```python
from build123d import *

# Parameters (mm, degrees)
BOSS_EXTRUDE1_DEPTH = 3
FILLET1_R           = 3
FILLET2_R           = 5
FILLET3_R           = 4
FILLET4_R           = 1
FILLET5_R           = 10


with BuildPart() as part:
    # Sketch2 → Boss-Extrude1 (new body)
    with BuildSketch(Plane(origin=(0, 0, 0), x_dir=(1, 0, 0), z_dir=(0, 1, 0))):
        with BuildLine():
            Line((104.861742338, 51.61), (96.285742338, 51.61))
            ThreePointArc((96.285742338, 51.61), (94.785742338, 50.11), (96.285742338, 48.61))
            Line((96.285742338, 48.61), (104.861742338, 48.61))
            Line((104.861742338, 48.61), (104.861742338, 42.36))
            Line((104.861742338, 42.36), (101.159535482, 30.341590159))
            ThreePointArc((101.159535482, 30.341590159), (102.15147179, 28.466473533), (104.026588416, 29.458409841))
            Line((104.026588416, 29.458409841), (107.0705594, 39.34))
            ThreePointArc((107.0705594, 39.34), (110.559148386, 33.719570051), (111.09, 27.125809175))
            Line((111.09, 27.125809175), (105.531161353, 18.360668643))
            ThreePointArc((105.531161353, 18.360668643), (84.319857644, 28.006827284), (67.651742338, 44.29))
            Line((67.651742338, 44.29), (61.935762488, 23.027584397))
            Line((61.935762488, 23.027584397), (57.13, 16.32))
            Line((57.13, 16.32), (49.95, 19.39))
            Line((49.95, 19.39), (25.830040494, 11.99))
            ThreePointArc((25.830040494, 11.99), (24.800734775, 10.253880031), (26.431506195, 9.064692331))
            ThreePointArc((26.431506195, 9.064692331), (36.664028635, 8.803570476), (46.46571567, 5.854056721))
            Line((46.46571567, 5.854056721), (45.9, 1.991540554))
            Line((45.9, 1.991540554), (41.660045255, 2.482673431))
            Line((41.660045255, 2.482673431), (38.9, -1.2))
            Line((38.9, -1.2), (27.015518097, 3.924692331))
            Line((27.015518097, 3.924692331), (20.16, 0))
            Line((20.16, 0), (0, 0))
            Line((0, 0), (0, 4.28))
            Line((0, 4.28), (8.255364291, 5.2))
            ThreePointArc((8.255364291, 5.2), (9.58, 6.856906829), (7.923093171, 8.181542538))
            Line((7.923093171, 8.181542538), (-3.121398875, 6.950714639))
            Line((-3.121398875, 6.950714639), (-7.499203077, 8.482641989))
            Line((-7.499203077, 8.482641989), (-11.827625236, 7.22158903))
            Line((-11.827625236, 7.22158903), (-19.255161489, 11.297641869))
            Line((-19.255161489, 11.297641869), (-23.205269456, 10.857431213))
            Line((-23.205269456, 10.857431213), (-22.269740859, 7.646334739))
            Line((-22.269740859, 7.646334739), (-24.812537217, 7.22158903))
            ThreePointArc((-24.812537217, 7.22158903), (-27.256062178, 10.796585791), (-27.5, 15.12))
            ThreePointArc((-27.5, 15.12), (-22.484233626, 16.792009689), (-17.704912147, 14.531121607))
            ThreePointArc((-17.704912147, 14.531121607), (-4.702395419, 12.521774189), (8.186937419, 15.161474421))
            Line((8.186937419, 15.161474421), (21.991482078, 21.019847276))
            Line((21.991482078, 21.019847276), (29.148159429, 28.986869108))
            Line((29.148159429, 28.986869108), (36.03, 31.378427725))
            Line((36.03, 31.378427725), (41.652863678, 73.662098134))
            ThreePointArc((41.652863678, 73.662098134), (47.001876481, 83.094401265), (57.4, 86.17))
            Line((57.4, 86.17), (89.772823478, 69.836247096))
            ThreePointArc((89.772823478, 69.836247096), (90.799785464, 67.40403524), (93.25912827, 66.443859006))
            ThreePointArc((93.25912827, 66.443859006), (102.166931279, 63.469413825), (107.0705594, 55.46))
            Line((107.0705594, 55.46), (104.861742338, 51.61))
        make_face()
    extrude(amount=BOSS_EXTRUDE1_DEPTH)

    # Fillet1
    fillet1_edges = [part.edges().sort_by_distance(p)[0] for p in [
        (46.46571567, 1.5, -5.854056721),
        (38.9, 1.5, 1.2),
        (20.16, 1.5, 0),
        (-27.5, 1.5, -15.12),
        (29.148159429, 1.5, -28.986869108),
        (89.772823478, 1.5, -69.836247096),
    ]]
    fillet(fillet1_edges, radius=FILLET1_R)

    # Fillet2
    fillet2_edges = [part.edges().sort_by_distance(p)[0] for p in [
        (104.861742338, 1.5, -42.36),
        (111.09, 1.5, -27.125809175),
        (105.531161353, 1.5, -18.360668643),
        (61.935762488, 1.5, -23.027584397),
        (49.95, 1.5, -19.39),
        (27.015518097, 1.5, -3.924692331),
    ]]
    fillet(fillet2_edges, radius=FILLET2_R)

    # Fillet3
    fillet3_edges = [part.edges().sort_by_distance(p)[0] for p in [
        (57.13, 1.5, -16.32),
        (-3.121398875, 1.5, -6.950714639),
        (-7.499203077, 1.5, -8.482641989),
        (-11.827625236, 1.5, -7.22158903),
        (-19.255161489, 1.5, -11.297641869),
        (36.03, 1.5, -31.378427725),
    ]]
    fillet(fillet3_edges, radius=FILLET3_R)

    # Fillet4
    fillet4_edges = [part.edges().sort_by_distance(p)[0] for p in [
        (45.9, 1.5, -1.991540554),
        (0, 1.5, 0),
        (-23.205269456, 1.5, -10.857431213),
        (-22.269740859, 1.5, -7.646334739),
        (-24.812537217, 1.5, -7.22158903),
    ]]
    fillet(fillet4_edges, radius=FILLET4_R)

    # Fillet5
    fillet5_edges = [part.edges().sort_by_distance(p)[0] for p in [
        (57.4, 1.5, -86.17),
    ]]
    fillet(fillet5_edges, radius=FILLET5_R)


solid = part.part
```
Input: part model. Units: mm. Frame: model coordinates. A direction names the side the tool comes from. Coordinates: 2 decimals unless noted, no trailing zeros. Write each loop counter-clockwise with the first axis right and the second up, starting at its lowest first coordinate (ties: lowest second). Pieces come first, ordered by that corner, then holes. Notation, with made-up numbers: (55.25, 28.5) -> (74.25, 28.5) arc R7 cw to (74.25, 37.5) -> close; hole circle Ø5 at (62, 47). An arc over 180 degrees is marked (long way). Answer as a JSON object with one key per item and string values.
1. Mould query, pull axis Z, two halves, no side actions, for faces 1 (the face through (-11.77, 1.521, -7.547)), 2 (the face through (9.583, 1.479, -6.824)), 3 (the face through (35.509, 1.521, -31.844)). Classes: released by +Z, released by -Z, zero draft, split by the parting line, or undercut.
Result set:
{"face 1": "released by +Z", "face 2": "undercut", "face 3": "released by -Z"}
2. Access query for faces 4 (the face through (73.81, 1.48, -77.89)), 5 (the face through (0, 1, -3)), 6 (the face through (105.98, 1.48, -53.56)), 7 (the face through (-15.679, 1.479, -9.335)), 8 (the face through (2.924, 1.479, -7.624)). Directions: +Z, -Z, +X, -X, +Y, -Y. A direction counts if a zero-diameter tool reaches every point of the face in a straight line with its end or side. Return the directions, or none.
Result set:
{"face 4": "-Z, +X, +Y, -Y", "face 5": "+Z, -X, +Y, -Y", "face 6": "+X, +Y, -Y", "face 7": "+Z, +Y, -Y", "face 8": "+Y, -Y"}
3. Section A-A on x = 55.5. Return the cut outline in (y, z), then the cut area to 3 significant figures.
Result set:
{"outline": "(0, -86.13) -> (3, -86.13) -> (3, -17.27) -> (0, -17.27) -> close", "area": "207 mm2"}
4. Section B-B on z = -50.11. Return the cut outline in (x, y), then the cut area to 3 significant figures.
Result set:
{"outline": "(38.52, 0) -> (94.79, 0) -> (94.79, 3) -> (38.52, 3) -> close", "area": "169 mm2"}
5. First-contact query: P1, Ø1.5, axis at x = 8, y = 1, coming from the +Z side; P2, Ø12, axis at x = 30.5, z = -63, coming from the +Y side; P3, Ø0.9, axis at y = 2, z = -47, coming from the +X side; P4, Ø1.5, axis at x = 61, y = 2.5, coming from the +Z side. Flat tips, straight axial feed; report the tip coordinate or a pass-through.
Result set:
{"P1": "stops at z = 0", "P2": "passes through", "P3": "stops at x = 104.86", "P4": "stops at z = -20.67"}
6. Material intervals for line 1 (X direction, y = 0.8, z = -32); line 2 (X direction, y = 1.7, z = -29); line 3 (Z direction, x = 17, y = 2.65), sorted ascending. Write a range as from..to.
Result set:
{"line 1": "x = 35.63..64.35, 79.06..101.67, 104.81..111.01", "line 2": "x = 29.35..63.54, 82.91..101.39, 103.79..111.26", "line 3": "z = -18.9..0"}
